Here's how the part is built. I have some questions about the finished solid (model axes, mm). Face numbers are marked on the shaded views. A direction names the side the tool comes from. Coordinates: 2 decimals unless noted, no trailing zeros. Order: outer loops, then holes, each group sorted by start corner. A loop starts at its lowest first (then second) coordinate and runs counter-clockwise, first axis right, second up.
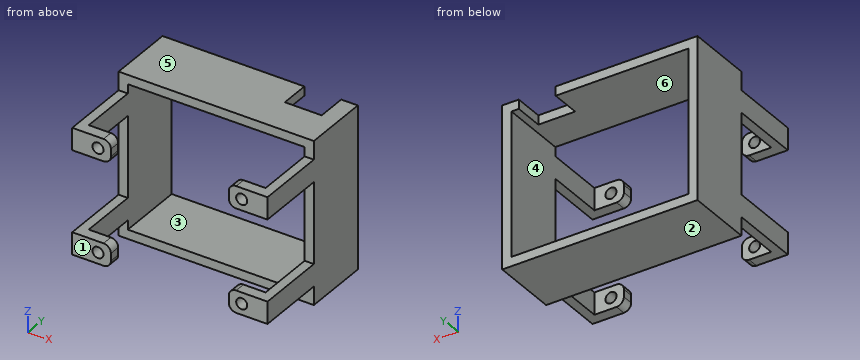
```python
from build123d import *

# Parameters (mm, degrees)
SKETCH_1_W          = 53
SKETCH_1_H          = 44
SKETCH_1_W_2        = 48
SKETCH_1_H_2        = 39
EXTRUDE_1_DEPTH     = 18
SKETCH_2_W          = 2.5
SKETCH_2_H          = 6
EXTRUDE_2_DEPTH     = 16
SKETCH_3_W          = 8
SKETCH_3_H          = 6
SKETCH_3_R          = 1.5
SKETCH_3_W_2        = 2.5
EXTRUDE_3_DEPTH     = 3
FILLET_1_R          = 2
SKETCH_4_W          = 10
SKETCH_4_H          = 8
CUT_EXTRUDE_1_DEPTH = 5


with BuildPart() as part:
    # 草图1 → 凸台-拉伸1 (new body)
    with BuildSketch(Plane(origin=(0, 0, 0), x_dir=(1, 0, 0), z_dir=(0, 1, 0))):
        Rectangle(SKETCH_1_W, SKETCH_1_H)
        Rectangle(SKETCH_1_W_2, SKETCH_1_H_2, mode=Mode.SUBTRACT)
    extrude(amount=EXTRUDE_1_DEPTH)

    # 草图2 → 凸台-拉伸2 (add)
    with BuildSketch(Plane.XZ):
        with Locations((25.25, 14)):
            Rectangle(SKETCH_2_W, SKETCH_2_H)
        with Locations((25.25, -14)):
            Rectangle(SKETCH_2_W, SKETCH_2_H)
        with Locations((-25.25, -14)):
            Rectangle(SKETCH_2_W, SKETCH_2_H)
        with Locations((-25.25, 14)):
            Rectangle(SKETCH_2_W, SKETCH_2_H)
    extrude(amount=EXTRUDE_2_DEPTH)

    # 草图3 → 凸台-拉伸3 (add)
    # profile 1 of 8: a face of its own
    with BuildSketch(Plane.XZ.offset(16)):
        with Locations((-20, 14)):
            Rectangle(SKETCH_3_W, SKETCH_3_H)
        with Locations(Location((-19.5, 14, 0), (0, 0, 270))):
            Circle(SKETCH_3_R, mode=Mode.SUBTRACT)
    # profile 2 of 8: a face of its own
    with BuildSketch(Plane.XZ.offset(16)):
        with Locations((-25.25, 14)):
            Rectangle(SKETCH_3_W_2, SKETCH_3_H)
    # profile 3 of 8: a face of its own
    with BuildSketch(Plane.XZ.offset(16)):
        with Locations((25.25, 14)):
            Rectangle(SKETCH_3_W_2, SKETCH_3_H)
    # profile 4 of 8: a face of its own
    with BuildSketch(Plane.XZ.offset(16)):
        with Locations((20, 14)):
            Rectangle(SKETCH_3_W, SKETCH_3_H)
        with Locations(Location((19.5, 14, 0), (0, 0, 270))):
            Circle(SKETCH_3_R, mode=Mode.SUBTRACT)
    # profile 5 of 8: a face of its own
    with BuildSketch(Plane.XZ.offset(16)):
        with Locations((20, -14)):
            Rectangle(SKETCH_3_W, SKETCH_3_H)
        with Locations(Location((19.5, -14, 0), (0, 0, 270))):
            Circle(SKETCH_3_R, mode=Mode.SUBTRACT)
    # profile 6 of 8: a face of its own
    with BuildSketch(Plane.XZ.offset(16)):
        with Locations((25.25, -14)):
            Rectangle(SKETCH_3_W_2, SKETCH_3_H)
    # profile 7 of 8: a face of its own
    with BuildSketch(Plane.XZ.offset(16)):
        with Locations((-25.25, -14)):
            Rectangle(SKETCH_3_W_2, SKETCH_3_H)
    # profile 8 of 8: a face of its own
    with BuildSketch(Plane.XZ.offset(16)):
        with Locations((-20, -14)):
            Rectangle(SKETCH_3_W, SKETCH_3_H)
        with Locations(Location((-19.5, -14, 0), (0, 0, 270))):
            Circle(SKETCH_3_R, mode=Mode.SUBTRACT)
    extrude(amount=EXTRUDE_3_DEPTH)

    # 圆角1
    fillet_1_edges = [part.edges().sort_by_distance(p)[0] for p in [
        (16, -17.5, -17),
        (16, -17.5, -11),
        (-16, -17.5, -17),
        (-16, -17.5, -11),
        (-16, -17.5, 17),
        (-16, -17.5, 11),
        (16, -17.5, 17),
        (16, -17.5, 11),
    ]]
    fillet(fillet_1_edges, radius=FILLET_1_R)

    # 草图4 → 切除-拉伸1 (cut)
    with BuildSketch(Plane.XY.offset(22)):
        with Locations((17, 14)):
            Rectangle(SKETCH_4_W, SKETCH_4_H)
    extrude(amount=-CUT_EXTRUDE_1_DEPTH, mode=Mode.SUBTRACT)


solid = part.part
```
Q1. I need wall thicknesses on L1, parallel to X at y = -17.4, z = -14; L2, parallel to Z at x = -19, y = -17; L3, parallel to X at y = 0.5, z = -19. Which ranges of each line are inside material? Lowest first, please.
Q2. Will these pins go through, and if not, where does the flat tip stop? pin 1 (2 mm diameter, centred on x = -25, z = -0.5, fed in from -Y); pin 2 (4 mm diameter, centred on x = -17.5, z = 16, fed in from +Y); pin 3 (2.5 mm diameter, centred on x = 23, y = -7, fed in from +Z).
Q3. We'd pull the mould along Z, two halves only. Please class the marked faces 1, 2 and 3: pulls with the +Z half, pulls with the -Z half, needs draft (parallel to the pull), parting line crosses it, or undercut.
Q4. If we section it at A-A on z = -9: Write out the boundary of the cut face in (x, y), then the cut area to 3 significant figures.
Q5. For the marked faces 4, 5 and 6, which set-ups out of +Z, -Z, +X, -X, +Y, -Y let a thin tool reach every point of the face, with its end or its side?
Q6. If we section it at B-B on x = -19.5: Write out the boundary of the cut face in (y, z), then the cut area to 3 significant figures.
Q7. If we section it at C-C on y = 9: Write out the boundary of the cut face in (x, z), then the cut area to 3 significant figures.
Q8. If we section it at D-D on z = -14: Write out the boundary of the cut face in (x, y).
Reply:
1. L1: x = -26.5 to -21, -18 to -16, 16 to 18, 21 to 26.5
1. L2: z = -17 to -15.41, -12.59 to -11, 11 to 12.59, 15.41 to 17
1. L3: x = -26.5 to -24, 24 to 26.5
2. pin 1: stops at y = 0
2. pin 2: stops at y = -16
2. pin 3: stops at z = 17
3. face 1: needs draft
3. face 2: pulls with the -Z half
3. face 3: undercut
4. outline: (-26.5, 0) - (-24, 0) - (-24, 18) - (-26.5, 18) - close; (24, 0) - (26.5, 0) - (26.5, 18) - (24, 18) - close
4. area: 90.0 mm2
5. face 4: +Y
5. face 5: +Z, +X, -X, +Y, -Y
5. face 6: +Y, -Y
6. outline: (-19, -17) - (-16, -17) - (-16, -15.5) - (-19, -15.5) - close; (-19, -12.5) - (-16, -12.5) - (-16, -11) - (-19, -11) - close; (-19, 11) - (-16, 11) - (-16, 12.5) - (-19, 12.5) - close; (-19, 15.5) - (-16, 15.5) - (-16, 17) - (-19, 17) - close; (0, -22) - (18, -22) - (18, -19.5) - (0, -19.5) - close; (0, 19.5) - (18, 19.5) - (18, 22) - (0, 22) - close
6. area: 108 mm2
7. outline: (-26.5, -22) - (26.5, -22) - (26.5, 22) - (-26.5, 22) - close; hole (-24, -19.5) - (24, -19.5) - (24, 19.5) - (-24, 19.5) - close
7. area: 460 mm2
8. outline: (-26.5, -19) - (-21, -19) - (-21, -16) - (-24, -16) - (-24, 18) - (-26.5, 18) - close; (-18, -19) - (-16, -19) - (-16, -16) - (-18, -16) - close; (16, -19) - (18, -19) - (18, -16) - (16, -16) - close; (21, -19) - (26.5, -19) - (26.5, 18) - (24, 18) - (24, -16) - (21, -16) - close
